Part model, mm, in its own coordinate system. Face numbers are marked on the shaded views. A direction names the side the tool comes from. Round coordinates to 2 decimals unless told otherwise and drop trailing zeros. Write each loop counter-clockwise with the first axis right and the second up, starting at its lowest first coordinate (ties: lowest second). Pieces come first, ordered by that corner, then holes.
1) Drill centre lines: L1, parallel to Y at x = 68.5, z = 2.7; L2, parallel to X at y = 18, z = 3.35; L3, parallel to Y at x = 68.5, z = 1.1. Where is each one in solid material? Low to high.
2) Which spindle directions (+Z, -Z, +X, -X, +Y, -Y) get a long thin tool onto all of the face, cutting with end or side? Do the marked faces 5 and 6. Say none if no direction does.
3) Saw through at A-A on z = 4. Count the separate pieces of the cut face and the enclosed holes in it, and give its area (3 significant figures).
4) Pull direction Y, two halves, no side cores. Call the marked faces 1, 2, 3 and 4: +Y half, -Y half, draft (parallel to the pull), parting line (faces both ways), or undercut.
5) Flat gauge pins, fed straight in: pin 1 (10 mm diameter, centred on x = 26.5, z = 10, fed in from -Y); pin 2 (3 mm diameter, centred on x = 68.5, y = 54.5, fed in from +Z); pin 3 (5 mm diameter, centred on x = 39.5, y = 16, fed in from +Z). Where does each tip first touch, or does it go through?
6) Saw through at B-B on y = 54. Write the cut outline in (x, z), and give its area (3 significant figures).
7) Saw through at D-D on z = 15.75. Write the cut outline in (x, y), and give its area (3 significant figures).
8) Saw through at C-C on x = 6.5. Write the cut outline in (y, z), and give its area (3 significant figures).
```python
from build123d import *

# Parameters (mm, degrees)
SKETCH_1_W          = 75
SKETCH_1_H          = 61
EXTRUDE_1_DEPTH     = 22
SKETCH_2_W          = 71
SKETCH_2_H          = 57
CUT_EXTRUDE_1_DEPTH = 100.146356464
SKETCH_3_W          = 75
SKETCH_3_H          = 61
EXTRUDE_2_DEPTH     = 2
SKETCH_4_R          = 3
EXTRUDE_3_DEPTH     = 5
SKETCH_5_R          = 1.1
CUT_EXTRUDE_2_DEPTH = 100.146356464


with BuildPart() as part:
    # 草图1 → 凸台-拉伸1 (new body)
    with BuildSketch(Plane.XY):
        with Locations((37.5, 30.5)):
            Rectangle(SKETCH_1_W, SKETCH_1_H)
    extrude(amount=EXTRUDE_1_DEPTH)

    # 草图2 → 切除-拉伸1 (cut, through all)
    with BuildSketch(Plane.XY):
        with Locations((37.5, 30.5)):
            Rectangle(SKETCH_2_W, SKETCH_2_H)
    extrude(amount=CUT_EXTRUDE_1_DEPTH, mode=Mode.SUBTRACT)

    # 草图3 → 凸台-拉伸2 (add)
    with BuildSketch(Plane.XY):
        with Locations((37.5, 30.5)):
            Rectangle(SKETCH_3_W, SKETCH_3_H)
    extrude(amount=EXTRUDE_2_DEPTH)

    # 草图4 → 凸台-拉伸3 (add)
    with BuildSketch(Plane.XY):
        with Locations(Location((6.5, 18, 0), (0, 0, 180))):
            Circle(SKETCH_4_R)
        with Locations(Location((68.5, 18, 0), (0, 0, 180))):
            Circle(SKETCH_4_R)
        with Locations(Location((6.5, 54, 0), (0, 0, 180))):
            Circle(SKETCH_4_R)
        with Locations(Location((68.5, 54, 0), (0, 0, 180))):
            Circle(SKETCH_4_R)
    extrude(amount=EXTRUDE_3_DEPTH)

    # 草图5 → 切除-拉伸2 (cut, through all)
    with BuildSketch(Plane.XY):
        with Locations((6.5, 18)):
            Circle(SKETCH_5_R)
        with Locations((68.5, 18)):
            Circle(SKETCH_5_R)
        with Locations((6.5, 54)):
            Circle(SKETCH_5_R)
        with Locations((68.5, 54)):
            Circle(SKETCH_5_R)
    extrude(amount=CUT_EXTRUDE_2_DEPTH, mode=Mode.SUBTRACT)


solid = part.part
```
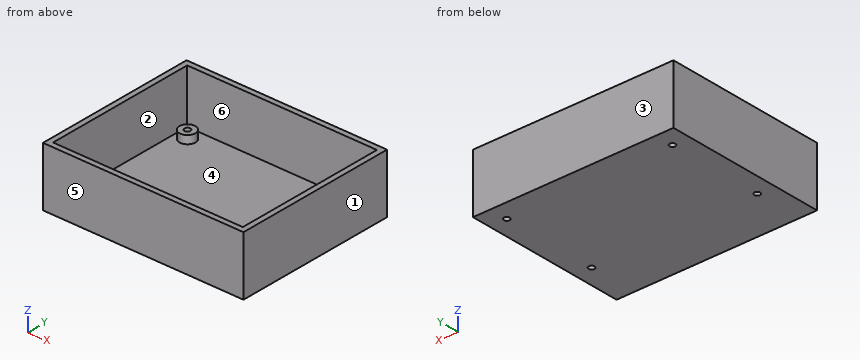
Completed:
1. L1: y = 0 to 2, 15 to 16.9, 19.1 to 21, 51 to 52.9, 55.1 to 57, 59 to 61
1. L2: x = 0 to 2, 3.5 to 5.4, 7.6 to 9.5, 65.5 to 67.4, 69.6 to 71.5, 73 to 75
1. L3: y = 0 to 16.9, 19.1 to 52.9, 55.1 to 61
2. face 5: +Z, -Z, +X, -X, -Y
2. face 6: +Z
3. separate pieces: 5
3. enclosed holes: 5
3. area: 626 mm2
4. face 1: draft
4. face 2: undercut
4. face 3: +Y half
4. face 4: undercut
5. pin 1: stops at y = 0
5. pin 2: stops at z = 5
5. pin 3: stops at z = 2
6. outline: (0, 0) - (5.4, 0) - (5.4, 5) - (3.5, 5) - (3.5, 2) - (2, 2) - (2, 22) - (0, 22) - close; (7.6, 0) - (67.4, 0) - (67.4, 5) - (65.5, 5) - (65.5, 2) - (9.5, 2) - (9.5, 5) - (7.6, 5) - close; (69.6, 0) - (75, 0) - (75, 22) - (73, 22) - (73, 2) - (71.5, 2) - (71.5, 5) - (69.6, 5) - close
6. area: 244 mm2
7. outline: (0, 0) - (75, 0) - (75, 61) - (0, 61) - close; hole (2, 2) - (73, 2) - (73, 59) - (2, 59) - close
7. area: 528 mm2
8. outline: (0, 0) - (16.9, 0) - (16.9, 5) - (15, 5) - (15, 2) - (2, 2) - (2, 22) - (0, 22) - close; (19.1, 0) - (52.9, 0) - (52.9, 5) - (51, 5) - (51, 2) - (21, 2) - (21, 5) - (19.1, 5) - close; (55.1, 0) - (61, 0) - (61, 22) - (59, 22) - (59, 2) - (57, 2) - (57, 5) - (55.1, 5) - close
8. area: 216 mm2
